Here's how the part is built. I have some questions about the finished solid (model axes, mm). Coordinates: 2 decimals unless noted, no trailing zeros. Write each loop counter-clockwise with the first axis right and the second up, starting at its lowest first coordinate (ties: lowest second). Pieces come first, ordered by that corner, then holes. Notation, with made-up numbers: (13.5, 30.25) - (38.5, 30.25) arc R13 ccw to (38.5, 36.25) - close; hole circle Ø11 at (1, 0). An arc over 180 degrees is marked (long way). Answer in a Markdown table with one row per item. Add a question column.
Item 1: Imagine slicing it at A-A (x = -9.5). Please give me the cut outline in (y, z).
Item 2: Imagine slicing it at B-B (y = 0.6). State how many separate pieces and enclosed holes the cut face has, plus the area to 3 significant figures.
Item 3: I'm going to push flat-ended pins straight in: pin 1 (0.5 mm diameter, centred on y = 1, z = 12, fed in from -X); pin 2 (5 mm diameter, centred on x = 35, z = 12.46, fed in from -Y); pin 3 (0.5 mm diameter, centred on y = 1, z = -12.5, fed in from +X); pin 4 (0.5 mm diameter, centred on y = 0.5, z = -13, fed in from -X). Where does each tip first touch, or does it pass through?
Item 4: If I drill on probe 1 along X at (y, z) = (0.8, 10.5); probe 2 along Z at (x, y) = (28, 0.8); probe 3 along Z at (x, y) = (4.5, 0.6), over which ranges is the centre line in solid material (lowest first)? Write a range as from..to.
from build123d import *

# Parameters (mm, degrees)
SKETCH_1_W          = 6
SKETCH_1_H          = 5
SKETCH_1_W_2        = 80
SKETCH_1_H_2        = 20
EXTRUDE_1_DEPTH     = 1.6
SKETCH_2_R          = 1.5
CUT_EXTRUDE_1_DEPTH = 43.74997076
FILLET_1_R          = 1
SKETCH_3_R          = 0.25
CUT_EXTRUDE_2_DEPTH = 43.74997076
FILLET_2_R          = 2


with BuildPart() as part:
    # Эскиз1 → Бобышка-Вытянуть1 (new body)
    with BuildSketch(Plane(origin=(0, 0, 0), x_dir=(1, 0, 0), z_dir=(0, 1, 0))):
        with Locations((-20, 12.5)):
            Rectangle(SKETCH_1_W, SKETCH_1_H)
        Rectangle(SKETCH_1_W_2, SKETCH_1_H_2)
        with Locations((20, 12.5)):
            Rectangle(SKETCH_1_W, SKETCH_1_H)
        with Locations((35, -12.5)):
            Rectangle(SKETCH_1_W, SKETCH_1_H)
        with Locations((5, -12.5)):
            Rectangle(SKETCH_1_W, SKETCH_1_H)
        with Locations((-5, -12.5)):
            Rectangle(SKETCH_1_W, SKETCH_1_H)
        with Locations((-35, -12.5)):
            Rectangle(SKETCH_1_W, SKETCH_1_H)
    extrude(amount=EXTRUDE_1_DEPTH)

    # Эскиз2 → Вырез-Вытянуть1 (cut, through all)
    with BuildSketch(Plane(origin=(0, 1.6, 0), x_dir=(1, 0, 0), z_dir=(0, 1, 0))):
        with Locations(Location((-20, 12.46, 0), (0, 0, 270))):
            Circle(SKETCH_2_R)
        with Locations(Location((-35, -12.46, 0), (0, 0, 270))):
            Circle(SKETCH_2_R)
        with Locations(Location((-5, -12.46, 0), (0, 0, 270))):
            Circle(SKETCH_2_R)
        with Locations(Location((5, -12.46, 0), (0, 0, 90))):
            Circle(SKETCH_2_R)
        with Locations(Location((35, -12.46, 0), (0, 0, 90))):
            Circle(SKETCH_2_R)
        with Locations(Location((20, 12.46, 0), (0, 0, 90))):
            Circle(SKETCH_2_R)
    extrude(amount=-CUT_EXTRUDE_1_DEPTH, mode=Mode.SUBTRACT)

    # Скругление1
    fillet_1_edges = [part.edges().sort_by_distance(p)[0] for p in [
        (32, 0, 12.5),
        (-23, 0.8, -15),
        (-17, 0.8, -15),
        (17, 0.8, -15),
        (23, 0.8, -15),
        (40, 0.8, 10),
        (38, 0.8, 15),
        (8, 0.8, 15),
        (2, 0.8, 15),
        (-2, 0.8, 15),
        (-8, 0.8, 15),
        (-32, 0.8, 15),
        (-38, 0.8, 15),
        (-40, 0.8, 10),
    ]]
    fillet(fillet_1_edges, radius=FILLET_1_R)

    # Эскиз3 → Вырез-Вытянуть2 (cut, through all)
    with BuildSketch(Plane(origin=(0, 1.6, 0), x_dir=(1, 0, 0), z_dir=(0, 1, 0))):
        with Locations((-23, 10)):
            Circle(SKETCH_3_R)
        with Locations(Location((-21.5, 10, 0), (0, 0, 270))):
            Circle(SKETCH_3_R)
        with Locations(Location((-20, 10, 0), (0, 0, 270))):
            Circle(SKETCH_3_R)
        with Locations(Location((-18.5, 10, 0), (0, 0, 270))):
            Circle(SKETCH_3_R)
        with Locations((-17, 10)):
            Circle(SKETCH_3_R)
        with Locations((-38, -10)):
            Circle(SKETCH_3_R)
        with Locations(Location((-36.5, -10, 0), (0, 0, 270))):
            Circle(SKETCH_3_R)
        with Locations(Location((-35, -10, 0), (0, 0, 270))):
            Circle(SKETCH_3_R)
        with Locations(Location((-33.5, -10, 0), (0, 0, 270))):
            Circle(SKETCH_3_R)
        with Locations((-32, -10)):
            Circle(SKETCH_3_R)
        with Locations((-8, -10)):
            Circle(SKETCH_3_R)
        with Locations(Location((-6.5, -10, 0), (0, 0, 270))):
            Circle(SKETCH_3_R)
        with Locations(Location((-5, -10, 0), (0, 0, 270))):
            Circle(SKETCH_3_R)
        with Locations(Location((-3.5, -10, 0), (0, 0, 270))):
            Circle(SKETCH_3_R)
        with Locations((-2, -10)):
            Circle(SKETCH_3_R)
        with Locations((2, -10)):
            Circle(SKETCH_3_R)
        with Locations(Location((3.5, -10, 0), (0, 0, 90))):
            Circle(SKETCH_3_R)
        with Locations(Location((5, -10, 0), (0, 0, 90))):
            Circle(SKETCH_3_R)
        with Locations(Location((6.5, -10, 0), (0, 0, 90))):
            Circle(SKETCH_3_R)
        with Locations((8, -10)):
            Circle(SKETCH_3_R)
        with Locations((32, -10)):
            Circle(SKETCH_3_R)
        with Locations(Location((33.5, -10, 0), (0, 0, 90))):
            Circle(SKETCH_3_R)
        with Locations(Location((35, -10, 0), (0, 0, 90))):
            Circle(SKETCH_3_R)
        with Locations(Location((36.5, -10, 0), (0, 0, 90))):
            Circle(SKETCH_3_R)
        with Locations((38, -10)):
            Circle(SKETCH_3_R)
        with Locations((17, 10)):
            Circle(SKETCH_3_R)
        with Locations(Location((18.5, 10, 0), (0, 0, 90))):
            Circle(SKETCH_3_R)
        with Locations(Location((20, 10, 0), (0, 0, 90))):
            Circle(SKETCH_3_R)
        with Locations(Location((21.5, 10, 0), (0, 0, 90))):
            Circle(SKETCH_3_R)
        with Locations((23, 10)):
            Circle(SKETCH_3_R)
    extrude(amount=-CUT_EXTRUDE_2_DEPTH, mode=Mode.SUBTRACT)

    # Скругление2
    fillet_2_edges = [part.edges().sort_by_distance(p)[0] for p in [
        (40, 0.8, -10),
        (-40, 0.8, -10),
    ]]
    fillet(fillet_2_edges, radius=FILLET_2_R)


solid = part.part
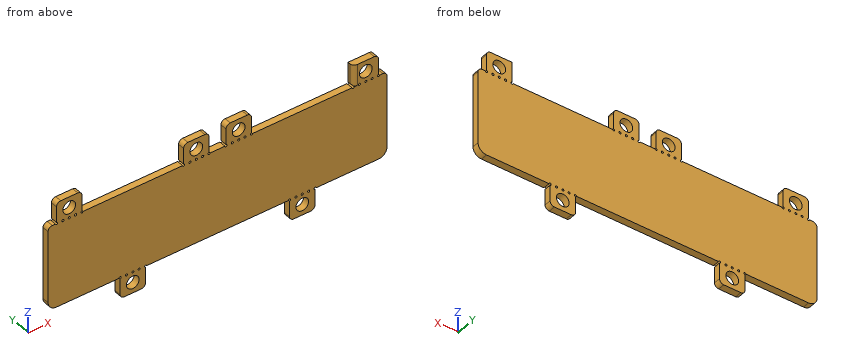
Here are the results:
| question | item | result |
|---|---|---|
| 1 | outline | (0, -10) - (1.6, -10) - (1.6, 10) - (0, 10) - close |
| 2 | separate pieces | 1 |
| 2 | enclosed holes | 24 |
| 2 | area | 1,730 mm2 |
| 3 | pin 1 | stops at x = -38 |
| 3 | pin 2 | stops at y = 0 |
| 3 | pin 3 | stops at x = 23 |
| 3 | pin 4 | stops at x = -23 |
| 4 | probe 1 | x = -38..-32, -8..-2, 2..8, 32.02..38 |
| 4 | probe 2 | z = -10..10 |
| 4 | probe 3 | z = -10..11.05, 13.87..15 |
